```python
from build123d import *

# Parameters (mm, degrees)
F0_W     = 75.241194
F0_H     = 61.288014
F0_R     = 9.804141
F1_DEPTH = 25.4
F2_DEPTH = 57.15
F4_DEPTH = 23.876


with BuildPart() as f1:
    # F0 (on Top) → F1 (new body)
    with BuildSketch(Plane.XY):
        with Locations((1.148045, 11.833709)):
            Rectangle(F0_W, F0_H)
        with Locations((0, 12.628511)):
            Circle(F0_R, mode=Mode.SUBTRACT)
    extrude(amount=F1_DEPTH)

    # F0 (on Top) → F2 (join)
    with BuildSketch(Plane.XY):
        with Locations((0, 12.628511)):
            Circle(F0_R)
    extrude(amount=F2_DEPTH)

    # F3 (on Right) → F4 (cut, symmetric)
    with BuildSketch(Plane.YZ):
        Polygon((-5.740232, 67.381494), (-4.327252, 36.295928), (35.589438, 67.381494), align=None)
    extrude(amount=F4_DEPTH, both=True, mode=Mode.SUBTRACT)


solid = f1.part
```
The listing builds one solid part. Answer for the finished solid, in the listing's coordinates (mm). A direction names the side the tool comes from. Give positions to 0.01 mm unless a question says otherwise; leave off trailing zeros. Order: outer loops, then holes, each group sorted by start corner. A loop starts at its lowest first (then second) coordinate and runs counter-clockwise, first axis right, second up.
Item 1: The part is cut by section A-A, the plane x = 0. Give the vertices of the cut face in (y, z), and give its area (3 significant figures).
From the geometry:
outline: (-18.81, 0) - (42.48, 0) - (42.48, 25.4) - (22.43, 25.4) - (22.43, 57.14) - (2.82, 41.87) - (2.82, 25.4) - (-18.81, 25.4) - close
area: 2,030 mm2
Item 2: The part is cut by section D-D, the plane y = 16. Give the vertices of the cut face in (x, z).
From the geometry:
outline: (-36.47, 0) - (38.77, 0) - (38.77, 25.4) - (9.21, 25.4) - (9.21, 52.13) - (-9.21, 52.13) - (-9.21, 25.4) - (-36.47, 25.4) - close
Item 3: Find the intervals of material crossed by probe 1 along Z at (x, y) = (-26.5, 1.5); probe 2 along X at (y, z) = (19.5, 50); probe 3 along X at (y, z) = (8, 28.5), in increasing order.
From the geometry:
probe 1: z = 0 to 25.4
probe 2: x = -6.99 to 6.99
probe 3: x = -8.64 to 8.64
Item 4: Given pin 1 Ø10 at (x, z) = (2.5, 34) entering from +Y; pin 2 Ø6 at (x, y) = (-1.5, 4.5) entering from +Z; pin 3 Ø5 at (x, z) = (11, 35.5) entering from +Y, each flat-ended and moving along its own axis, determine where each tip first touches the part or whether it passes through.
From the geometry:
pin 1: stops at y = 22.43
pin 2: stops at z = 45.51
pin 3: stops at y = 17.51
Item 5: The part is cut by section B-B, the plane y = -11. Give the vertices of the cut face in (x, z), and give its area (3 significant figures).
From the geometry:
outline: (-36.47, 0) - (38.77, 0) - (38.77, 25.4) - (-36.47, 25.4) - close
area: 1,910 mm2
Item 6: The part is cut by section C-C, the plane z = 35.5. Give the vertices of the cut face in (x, y), and give its area (3 significant figures).
From the geometry:
outline: circle Ø19.61 at (0, 12.63)
area: 302 mm2
Item 7: Which of the six approach directions +Z, -Z, +X, -X, +Y, -Y give full straight-line access (tool end or side, diameter ignored) to faces 1 (the face through (38.769, 11, 13)), 2 (the face through (-1.28, 22.35, 37.59))?
From the geometry:
face 1: +Z, -Z, +X, +Y, -Y
face 2: +Z
